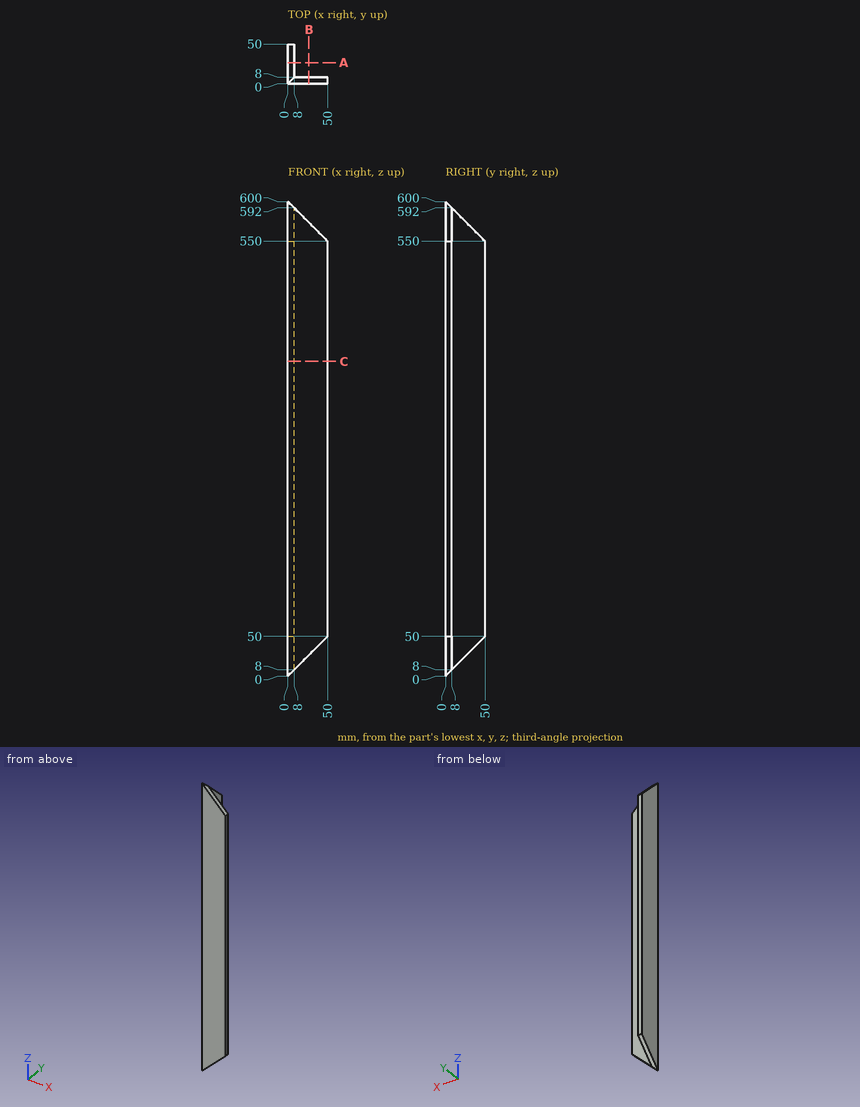
Verification items for this drawing (mm, ordinates from the low corner). Coordinates: 2 decimals unless noted, no trailing zeros. Write each loop counter-clockwise with the first axis right and the second up, starting at its lowest first coordinate (ties: lowest second). Pieces come first, ordered by that corner, then holes. Notation, with made-up numbers: (80.25, 51) -> (118.25, 51) arc R20 ccw to (118.25, 74) -> close; hole circle Ø5 at (27, 8.25). An arc over 180 degrees is marked (long way). One line per item, written item: value. Start each with the question number.
Q1. Cross-section at C-C on z = 398. Enter the section's corners in (x, y).
Q2. Cross-section at A-A on y = 26.5. Enter the section's corners in (x, z), and give its area (3 significant figures).
Q3. Thickness scan on L1, parallel to X at y = 20, z = 548; L2, parallel to Z at x = 37, y = 5. Record the ranges inside material, lowest first. Write a range as from..to.
Q4. Go/stop test with flat-tipped pins: P1, Ø2, axis at x = 27, z = 102.5, coming from the +Y side; P2, Ø2, axis at y = 38, z = 535.5, coming from the +X side. Record where each tip stops, or that it passes through.
Checked values:
1. outline: (0, 0) -> (50, 0) -> (50, 8) -> (8, 8) -> (8, 50) -> (0, 50) -> close
2. outline: (0, 26.5) -> (8, 26.5) -> (8, 573.5) -> (0, 573.5) -> close
2. area: 4,380 mm²
3. L1: x = 0..8
3. L2: z = 37..563
4. P1: stops at y = 8
4. P2: stops at x = 8
